Design review of the part built by this model. Coordinates are the model's own, in mm. Coordinates: 2 decimals unless noted, no trailing zeros. Answer as a JSON object with one key per item and string values. Group by question number.
1. Consider section A-A (y = 226.5). Count the separate pieces of the cut face and the enclosed holes in it, then the cut area to 3 significant figures.
2. Insertion check: pin 1 (1.3 mm diameter, centred on y = 265, z = -9.5, fed in from -X); pin 2 (1.3 mm diameter, centred on x = 31, y = 291.5, fed in from -Z); pin 3 (1.3 mm diameter, centred on y = 479, z = -10.5, fed in from +X). Each pin has a flat end and moves straight along its axis. Give the tip position at first contact, or say it passes through.
3. To check wall thickness, follow probe 1 along X at (y, z) = (407.5, -10); probe 2 along X at (y, z) = (491, -18.75); probe 3 along Z at (x, y) = (18, 174). State the ranges of each line that lie inside material, in increasing order.
from build123d import *

# Parameters (mm, degrees)
SKETCH1_R           = 2.15
BOSS_EXTRUDE1_DEPTH = 750


with BuildPart() as part:
    # Sketch1 → Boss-Extrude1 (new body)
    with BuildSketch(Plane(origin=(0, 0, 0), x_dir=(1, 0, 0), z_dir=(0, 1, 0))):
        with BuildLine():
            Line((7.5, 20), (7.5, 18.5))
            Line((7.5, 18.5), (5.014213562, 18.5))
            ThreePointArc((5.014213562, 18.5), (4.09033403, 17.882683432), (4.307106781, 16.792893219))
            Line((4.307106781, 16.792893219), (7.207106781, 13.892893219))
            ThreePointArc((7.207106781, 13.892893219), (7.53153013, 13.676120467), (7.914213562, 13.6))
            Line((7.914213562, 13.6), (12.085786438, 13.6))
            ThreePointArc((12.085786438, 13.6), (12.46846987, 13.676120467), (12.792893219, 13.892893219))
            Line((12.792893219, 13.892893219), (15.692893219, 16.792893219))
            ThreePointArc((15.692893219, 16.792893219), (15.90966597, 17.882683432), (14.985786438, 18.5))
            Line((14.985786438, 18.5), (12.5, 18.5))
            Line((12.5, 18.5), (12.5, 20))
            Line((12.5, 20), (27.5, 20))
            Line((27.5, 20), (27.5, 18.5))
            Line((27.5, 18.5), (25.014213562, 18.5))
            ThreePointArc((25.014213562, 18.5), (24.09033403, 17.882683432), (24.307106781, 16.792893219))
            Line((24.307106781, 16.792893219), (27.207106781, 13.892893219))
            ThreePointArc((27.207106781, 13.892893219), (27.53153013, 13.676120467), (27.914213562, 13.6))
            Line((27.914213562, 13.6), (32.085786438, 13.6))
            ThreePointArc((32.085786438, 13.6), (32.46846987, 13.676120467), (32.792893219, 13.892893219))
            Line((32.792893219, 13.892893219), (35.692893219, 16.792893219))
            ThreePointArc((35.692893219, 16.792893219), (35.90966597, 17.882683432), (34.985786438, 18.5))
            Line((34.985786438, 18.5), (32.5, 18.5))
            Line((32.5, 18.5), (32.5, 20))
            Line((32.5, 20), (47.5, 20))
            Line((47.5, 20), (47.5, 18.5))
            Line((47.5, 18.5), (45.014213562, 18.5))
            ThreePointArc((45.014213562, 18.5), (44.09033403, 17.882683432), (44.307106781, 16.792893219))
            Line((44.307106781, 16.792893219), (47.207106781, 13.892893219))
            ThreePointArc((47.207106781, 13.892893219), (47.53153013, 13.676120467), (47.914213562, 13.6))
            Line((47.914213562, 13.6), (52.085786438, 13.6))
            ThreePointArc((52.085786438, 13.6), (52.46846987, 13.676120467), (52.792893219, 13.892893219))
            Line((52.792893219, 13.892893219), (55.692893219, 16.792893219))
            ThreePointArc((55.692893219, 16.792893219), (55.90966597, 17.882683432), (54.985786438, 18.5))
            Line((54.985786438, 18.5), (52.5, 18.5))
            Line((52.5, 18.5), (52.5, 20))
            Line((52.5, 20), (59, 20))
            ThreePointArc((59, 20), (59.707106781, 19.707106781), (60, 19))
            Line((60, 19), (60, 12.5))
            Line((60, 12.5), (58.5, 12.5))
            Line((58.5, 12.5), (58.5, 14.985786438))
            ThreePointArc((58.5, 14.985786438), (57.882683432, 15.90966597), (56.792893219, 15.692893219))
            Line((56.792893219, 15.692893219), (53.892893219, 12.792893219))
            ThreePointArc((53.892893219, 12.792893219), (53.676120467, 12.46846987), (53.6, 12.085786438))
            Line((53.6, 12.085786438), (53.6, 7.914213562))
            ThreePointArc((53.6, 7.914213562), (53.676120467, 7.53153013), (53.892893219, 7.207106781))
            Line((53.892893219, 7.207106781), (56.792893219, 4.307106781))
            ThreePointArc((56.792893219, 4.307106781), (57.882683432, 4.09033403), (58.5, 5.014213562))
            Line((58.5, 5.014213562), (58.5, 7.5))
            Line((58.5, 7.5), (60, 7.5))
            Line((60, 7.5), (60, 1))
            ThreePointArc((60, 1), (59.707106781, 0.292893219), (59, 0))
            Line((59, 0), (52.5, 0))
            Line((52.5, 0), (52.5, 1.5))
            Line((52.5, 1.5), (54.985786438, 1.5))
            ThreePointArc((54.985786438, 1.5), (55.90966597, 2.117316568), (55.692893219, 3.207106781))
            Line((55.692893219, 3.207106781), (52.792893219, 6.107106781))
            ThreePointArc((52.792893219, 6.107106781), (52.46846987, 6.323879533), (52.085786438, 6.4))
            Line((52.085786438, 6.4), (47.914213562, 6.4))
            ThreePointArc((47.914213562, 6.4), (47.53153013, 6.323879533), (47.207106781, 6.107106781))
            Line((47.207106781, 6.107106781), (44.307106781, 3.207106781))
            ThreePointArc((44.307106781, 3.207106781), (44.09033403, 2.117316568), (45.014213562, 1.5))
            Line((45.014213562, 1.5), (47.5, 1.5))
            Line((47.5, 1.5), (47.5, 0))
            Line((47.5, 0), (32.5, 0))
            Line((32.5, 0), (32.5, 1.5))
            Line((32.5, 1.5), (34.985786438, 1.5))
            ThreePointArc((34.985786438, 1.5), (35.90966597, 2.117316568), (35.692893219, 3.207106781))
            Line((35.692893219, 3.207106781), (32.792893219, 6.107106781))
            ThreePointArc((32.792893219, 6.107106781), (32.46846987, 6.323879533), (32.085786438, 6.4))
            Line((32.085786438, 6.4), (27.914213562, 6.4))
            ThreePointArc((27.914213562, 6.4), (27.53153013, 6.323879533), (27.207106781, 6.107106781))
            Line((27.207106781, 6.107106781), (24.307106781, 3.207106781))
            ThreePointArc((24.307106781, 3.207106781), (24.09033403, 2.117316568), (25.014213562, 1.5))
            Line((25.014213562, 1.5), (27.5, 1.5))
            Line((27.5, 1.5), (27.5, 0))
            Line((27.5, 0), (12.5, 0))
            Line((12.5, 0), (12.5, 1.5))
            Line((12.5, 1.5), (14.985786438, 1.5))
            ThreePointArc((14.985786438, 1.5), (15.90966597, 2.117316568), (15.692893219, 3.207106781))
            Line((15.692893219, 3.207106781), (12.792893219, 6.107106781))
            ThreePointArc((12.792893219, 6.107106781), (12.46846987, 6.323879533), (12.085786438, 6.4))
            Line((12.085786438, 6.4), (7.914213562, 6.4))
            ThreePointArc((7.914213562, 6.4), (7.53153013, 6.323879533), (7.207106781, 6.107106781))
            Line((7.207106781, 6.107106781), (4.307106781, 3.207106781))
            ThreePointArc((4.307106781, 3.207106781), (4.09033403, 2.117316568), (5.014213562, 1.5))
            Line((5.014213562, 1.5), (7.5, 1.5))
            Line((7.5, 1.5), (7.5, 0))
            Line((7.5, 0), (1, 0))
            ThreePointArc((1, 0), (0.292893219, 0.292893219), (0, 1))
            Line((0, 1), (0, 7.5))
            Line((0, 7.5), (1.5, 7.5))
            Line((1.5, 7.5), (1.5, 5.014213562))
            ThreePointArc((1.5, 5.014213562), (2.117316568, 4.09033403), (3.207106781, 4.307106781))
            Line((3.207106781, 4.307106781), (6.107106781, 7.207106781))
            ThreePointArc((6.107106781, 7.207106781), (6.323879533, 7.53153013), (6.4, 7.914213562))
            Line((6.4, 7.914213562), (6.4, 12.085786438))
            ThreePointArc((6.4, 12.085786438), (6.323879533, 12.46846987), (6.107106781, 12.792893219))
            Line((6.107106781, 12.792893219), (3.207106781, 15.692893219))
            ThreePointArc((3.207106781, 15.692893219), (2.117316568, 15.90966597), (1.5, 14.985786438))
            Line((1.5, 14.985786438), (1.5, 12.5))
            Line((1.5, 12.5), (0, 12.5))
            Line((0, 12.5), (0, 19))
            ThreePointArc((0, 19), (0.292893219, 19.707106781), (1, 20))
            Line((1, 20), (7.5, 20))
        make_face()
        with Locations(Location((10, 10, 0), (0, 0, 270))):
            Circle(SKETCH1_R, mode=Mode.SUBTRACT)
        with Locations(Location((30, 10, 0), (0, 0, 270))):
            Circle(SKETCH1_R, mode=Mode.SUBTRACT)
        with Locations(Location((50, 10, 0), (0, 0, 270))):
            Circle(SKETCH1_R, mode=Mode.SUBTRACT)
        with BuildLine():
            Line((19.292893219, 18.192893219), (13.892893219, 12.792893219))
            ThreePointArc((13.892893219, 12.792893219), (13.676120467, 12.46846987), (13.6, 12.085786438))
            Line((13.6, 12.085786438), (13.6, 7.914213562))
            ThreePointArc((13.6, 7.914213562), (13.676120467, 7.53153013), (13.892893219, 7.207106781))
            Line((13.892893219, 7.207106781), (19.292893219, 1.807106781))
            ThreePointArc((19.292893219, 1.807106781), (20, 1.514213562), (20.707106781, 1.807106781))
            Line((20.707106781, 1.807106781), (26.107106781, 7.207106781))
            ThreePointArc((26.107106781, 7.207106781), (26.323879533, 7.53153013), (26.4, 7.914213562))
            Line((26.4, 7.914213562), (26.4, 12.085786438))
            ThreePointArc((26.4, 12.085786438), (26.323879533, 12.46846987), (26.107106781, 12.792893219))
            Line((26.107106781, 12.792893219), (20.707106781, 18.192893219))
            ThreePointArc((20.707106781, 18.192893219), (20, 18.485786438), (19.292893219, 18.192893219))
        make_face(mode=Mode.SUBTRACT)
        with BuildLine():
            Line((33.6, 12.085786438), (33.6, 7.914213562))
            ThreePointArc((33.6, 7.914213562), (33.676120467, 7.53153013), (33.892893219, 7.207106781))
            Line((33.892893219, 7.207106781), (39.292893219, 1.807106781))
            ThreePointArc((39.292893219, 1.807106781), (40, 1.514213562), (40.707106781, 1.807106781))
            Line((40.707106781, 1.807106781), (46.107106781, 7.207106781))
            ThreePointArc((46.107106781, 7.207106781), (46.323879533, 7.53153013), (46.4, 7.914213562))
            Line((46.4, 7.914213562), (46.4, 12.085786438))
            ThreePointArc((46.4, 12.085786438), (46.323879533, 12.46846987), (46.107106781, 12.792893219))
            Line((46.107106781, 12.792893219), (40.707106781, 18.192893219))
            ThreePointArc((40.707106781, 18.192893219), (40, 18.485786438), (39.292893219, 18.192893219))
            Line((39.292893219, 18.192893219), (33.892893219, 12.792893219))
            ThreePointArc((33.892893219, 12.792893219), (33.676120467, 12.46846987), (33.6, 12.085786438))
        make_face(mode=Mode.SUBTRACT)
    extrude(amount=BOSS_EXTRUDE1_DEPTH)


solid = part.part
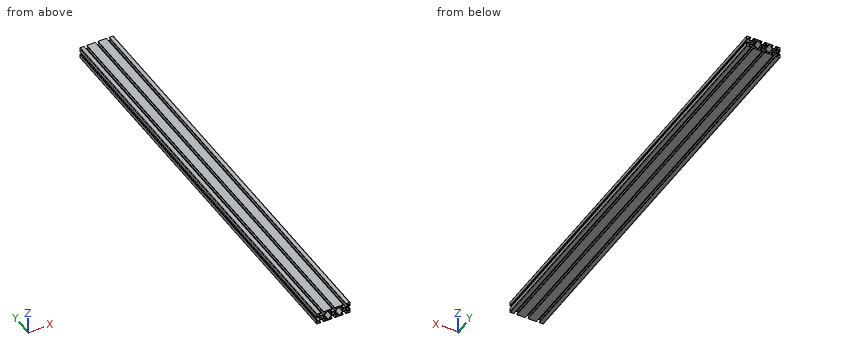
Findings below:
{
 "1": {"separate pieces": "1", "enclosed holes": "5", "area": "437 mm^2"},
 "2": {"pin 1": "stops at x = 6.4", "pin 2": "stops at z = -13.6", "pin 3": "stops at x = 53.6"},
 "3": {"probe 1": "x = 6.4 to 7.85, 12.15 to 13.6, 26.4 to 27.85, 32.15 to 33.6, 46.4 to 47.85, 52.15 to 53.6", "probe 2": "x = 0 to 7.5, 12.5 to 27.5, 32.5 to 47.5, 52.5 to 60", "probe 3": "z = -20 to -16.9, -3.1 to 0"}
}
